```python
from build123d import *

# Parameters (mm, degrees)
SKETCH1_W                 = 76
SKETCH1_H                 = 55.5
BOSS_EXTRUDE1_DEPTH       = 4
BOSS_EXTRUDE2_DEPTH       = 2.5
F_4_0MM_DOWEL_HOLE1_D     = 4
F_4_0MM_DOWEL_HOLE1_DEPTH = 6.5


with BuildPart() as part:
    # Sketch1 → Boss-Extrude1 (new body)
    with BuildSketch(Plane.XY):
        with Locations((-0.361045131, -5.590855107)):
            Rectangle(SKETCH1_W, SKETCH1_H)
    extrude(amount=BOSS_EXTRUDE1_DEPTH)

    # Sketch2 → Boss-Extrude2 (add)
    with BuildSketch(Plane.XY.offset(4)):
        Polygon((-38.361045131, 22.159144893), (37.638954869, 22.159144893), (37.638954869, 16.159144893), (37.638954869, 8.159144893), (37.638954869, -14.840855107), (33.638954869, -14.840855107), (33.638954869, 8.159144893), (31.638954869, 8.159144893), (31.638954869, 16.159144893), (-33.361045131, 16.159144893), (-33.361045131, -26.340855107), (-30.361045131, -29.340855107), (30.638954869, -29.340855107), (30.638954869, -21.340855107), (37.638954869, -21.340855107), (37.638954869, -29.340855107), (37.638954869, -33.340855107), (-33.361045131, -33.340855107), (-38.361045131, -33.340855107), (-38.361045131, 16.159144893), align=None)
    extrude(amount=BOSS_EXTRUDE2_DEPTH)

    # Ø4.0mm Dowel Hole1
    with Locations(Plane.XY.offset(6.5)):
        with Locations((-34.361045131, 18.159144893), (33.638954869, 18.159144893), (33.638954869, -29.340855107), (-34.361045131, -29.340855107)):
            Hole(F_4_0MM_DOWEL_HOLE1_D / 2, depth=F_4_0MM_DOWEL_HOLE1_DEPTH)


solid = part.part
```
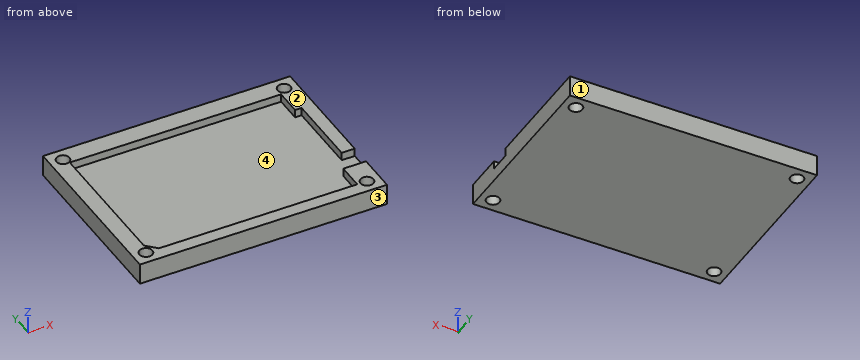
Geometry check sheet. Reference: the model listing, model coordinates, mm. Face numbers are marked on the shaded views. Coordinates: 2 decimals unless noted, no trailing zeros. Write each loop counter-clockwise with the first axis right and the second up, starting at its lowest first coordinate (ties: lowest second). Pieces come first, ordered by that corner, then holes. Notation, with made-up numbers: (-29.75, 51.25) -> (0.25, 51.25) arc R20 cw to (0.25, 88.25) -> close; hole circle Ø7 at (-25.5, 78). An arc over 180 degrees is marked (long way). Use CSV: the item, a comma, the result in double quotes. Start each with the question number.
Item 1: Depth check by flat-ended pin: pin 1 Ø2.5 at (x, y) = (33.64, -29.34) entering from -Z; pin 2 Ø1 at (x, y) = (23.5, -1.5) entering from +Z. Enter the tip coordinate at first touch or a pass-through.
Item 2: Mould release check, pull along Y, two halves, no side actions. Record for the marked faces 1, 2, 3 and 4: released by +Y, released by -Y, zero draft, split by the parting line, or undercut.
Item 3: Cross-section at A-A, the plane z = 5.5. Record the cut outline in (x, y), plus the area to 3 significant figures.
Item 4: Cross-section at C-C, the plane x = -19. Record the cut outline in (y, z).
Item 5: Cross-section at B-B, the plane y = -11. Record the cut outline in (x, z).
Item 6: Thickness scan on line 1 (X direction, y = -8.5, z = 6); line 2 (X direction, y = 11, z = 5.75); line 3 (Y direction, x = -25, z = 4.25). Record the ranges inside material, lowest first.
Item 7: Cross-section at D-D, the plane y = -18.5. Record the cut outline in (x, z), plus the area to 4 significant figures.
Answers:
1,pin 1,"through"
1,pin 2,"z = 4"
2,face 1,"released by +Y"
2,face 2,"zero draft"
2,face 3,"released by -Y"
2,face 4,"undercut"
3,outline,"(-38.36, -33.34) -> (37.64, -33.34) -> (37.64, -21.34) -> (30.64, -21.34) -> (30.64, -29.34) -> (-30.36, -29.34) -> (-33.36, -26.34) -> (-33.36, 16.16) -> (31.64, 16.16) -> (31.64, 8.16) -> (33.64, 8.16) -> (33.64, -14.84) -> (37.64, -14.84) -> (37.64, 22.16) -> (-38.36, 22.16) -> close; hole circle Ø4 at (-34.36, -29.34); hole circle Ø4 at (-34.36, 18.16); hole circle Ø4 at (33.64, -29.34); hole circle Ø4 at (33.64, 18.16)"
3,area,"1,140 mm^2"
4,outline,"(-33.34, 0) -> (22.16, 0) -> (22.16, 6.5) -> (16.16, 6.5) -> (16.16, 4) -> (-29.34, 4) -> (-29.34, 6.5) -> (-33.34, 6.5) -> close"
5,outline,"(-38.36, 0) -> (37.64, 0) -> (37.64, 6.5) -> (33.64, 6.5) -> (33.64, 4) -> (-33.36, 4) -> (-33.36, 6.5) -> (-38.36, 6.5) -> close"
6,line 1,"-38.36 to -33.36, 33.64 to 37.64"
6,line 2,"-38.36 to -33.36, 31.64 to 37.64"
6,line 3,"-33.34 to -29.34, 16.16 to 22.16"
7,outline,"(-38.36, 0) -> (37.64, 0) -> (37.64, 4) -> (-33.36, 4) -> (-33.36, 6.5) -> (-38.36, 6.5) -> close"
7,area,"316.5 mm^2"
